Design review of the part built by this model. Coordinates are the model's own, in mm. Face numbers are marked on the shaded views. Coordinates: 2 decimals unless noted, no trailing zeros. Write each loop counter-clockwise with the first axis right and the second up, starting at its lowest first coordinate (ties: lowest second). Pieces come first, ordered by that corner, then holes. Notation, with made-up numbers: M 72.5,6.25 L 111.5,6.25 A34 cw 111.5,36.25 Z; hole C 28,25 d3. An arc over 180 degrees is marked long. Return JSON: item names as keys, results as strings. Group by question number.
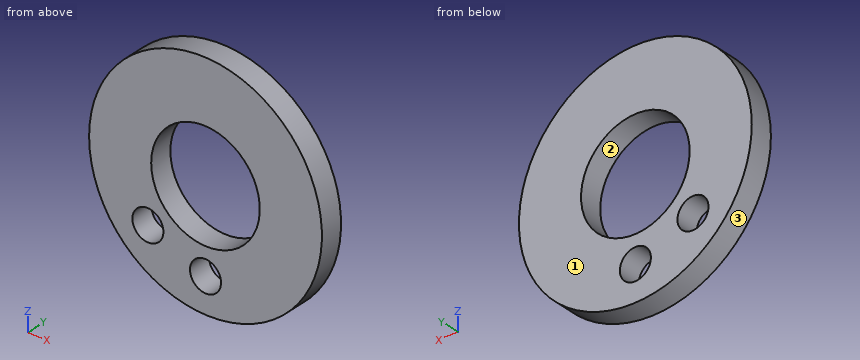
Autodesk Inventor part; units mm, degrees
ref_plane "YZ Plane" through (0, 0, 0) normal (1, 0, 0) x (0, 1, 0)
ref_plane "XZ Plane" through (0, 0, 0) normal (0, 1, 0) x (-1, 0, 0)
ref_plane "XY Plane" through (0, 0, 0) normal (0, 0, 1) x (1, 0, 0)
sketch "Sketch1" plane through (0, 0, 0) normal (0, 1, 0) x (-1, 0, 0)
  circle A0 centre (0, 0) radius 15
  circle A1 centre (0, 0) radius 7
  dimension "d0" = 30
  dimension "d1" = 14
  dimension "d6" = 0
extrude "Extrusion1" add sketch "Sketch1" along normal blind 3
sketch "Sketch2" plane through (0, 3, 0) normal (0, 1, 0) x (1, 0, 0)
  circle A0 centre (0, 0) radius 15
  line L0 (0, 0) -> (0, 10.5) construction
  circle A1 centre (0, 0) radius 10.5 construction
  line L1 (0, 0) -> (10.5, 0) construction
  dimension "d14" = 21
  dimension "d25" = 90
hole "Hole1" at (0, 3, -10.5) direction (0, -1, 0) diameter 4 end through all
pattern_circular "Circular Pattern2" count 2 over 45 about axis through (0, 0, 0) along (0, 1, 0) of "Hole1"
properties part number "OringProbe_ring_pipe_adapter_4mm_version" material "Stainless Steel, 440C"
Item 1: Add section D-D (y = 1.1). Write out the cut boundary in (x, z), plus the area to 3 significant figures.
Item 2: Add section A-A (z = 0). Write out the cut boundary in (x, y), plus the area to 3 significant figures.
Item 3: Add section C-C (x = -8.75). Write out the cut boundary in (y, z).
Item 4: For pin 1 (1.5 mm diameter, centred on y = 1.5, z = 4.5, fed in from -X), flat-tipped, find the tip position at first contact; note if it passes through.
Item 5: For line 1 (Z direction, x = 0, y = 1.7); line 2 (X direction, y = 2.8, z = 0.25); line 3 (Z direction, x = 0.5, y = 1.3), list the stretches that pass through material, from the lowest coordinate up.
Item 6: Add section B-B (x = 0). Write out the cut boundary in (y, z), plus the area to 3 significant figures.
Item 7: The part is to be moulded in two halves that separate along Z. For the marked faces 1, 2 and 3, say which applies: pulls with the +Z half, pulls with the -Z half, needs draft (parallel to the pull), parting line crosses it, or undercut.
Geometry check:
{
 "1": {"outline": "C 0,0 d30; hole C -7.42,-7.42 d4; hole C 0,0 d14; hole C 0,-10.5 d4", "area": "528 mm^2"},
 "2": {"outline": "M -15,0 L -7,0 L -7,3 L -15,3 Z; M 7,0 L 15,0 L 15,3 L 7,3 Z", "area": "48.0 mm^2"},
 "3": {"outline": "M 0,-12.18 L 3,-12.18 L 3,-8.92 L 0,-8.92 Z; M 0,-5.93 L 3,-5.93 L 3,12.18 L 0,12.18 Z"},
 "4": {"pin 1": "x = -14.52"},
 "5": {"line 1": "-15 to -12.5, -8.5 to -7, 7 to 15", "line 2": "-15 to -7, 7 to 15", "line 3": "-14.99 to -12.44, -8.56 to -6.98, 6.98 to 14.99"},
 "6": {"outline": "M 0,-15 L 3,-15 L 3,-12.5 L 0,-12.5 Z; M 0,-8.5 L 3,-8.5 L 3,-7 L 0,-7 Z; M 0,7 L 3,7 L 3,15 L 0,15 Z", "area": "36.0 mm^2"},
 "7": {"face 1": "needs draft", "face 2": "undercut", "face 3": "parting line crosses it"}
}
